from build123d import *

# Parameters (mm, degrees)
ESQUISSE1_W                                        = 65
ESQUISSE1_H                                        = 82
BOSS_EXTRU_1_DEPTH                                 = 10
CHAMBRAGE_POUR_VIS_T_TE_HEXAGONALE_M51_D           = 5.5
CHAMBRAGE_POUR_VIS_T_TE_HEXAGONALE_M51_CBORE_D     = 10
CHAMBRAGE_POUR_VIS_T_TE_HEXAGONALE_M51_CBORE_DEPTH = 7
TROU_TARAUD_M42_D                                  = 3.3
TROU_TARAUD_M42_DEPTH                              = 11.5
TROU_TARAUD_M42_TIP                                = 0.991420021
TROUS_DE_CENTRAGE_4_0MMTRANSITIONAL_1_D            = 4
TROUS_DE_CENTRAGE_4_0MMTRANSITIONAL_1_DEPTH        = 8
TROUS_DE_CENTRAGE_4_0MMTRANSITIONAL_1_TIP          = 1.154700538
TROU_TARAUD_M61_D                                  = 5


with BuildPart() as part:
    # Esquisse1 → Boss.-Extru.1 (new body)
    with BuildSketch(Plane.XY):
        Rectangle(ESQUISSE1_W, ESQUISSE1_H)
    extrude(amount=BOSS_EXTRU_1_DEPTH)

    # Chambrage pour vis à tête hexagonale M51 (through all)
    with Locations(Plane.XY.offset(10)):
        with Locations((10.25, 10), (-9.75, -10)):
            CounterBoreHole(CHAMBRAGE_POUR_VIS_T_TE_HEXAGONALE_M51_D / 2, CHAMBRAGE_POUR_VIS_T_TE_HEXAGONALE_M51_CBORE_D / 2, CHAMBRAGE_POUR_VIS_T_TE_HEXAGONALE_M51_CBORE_DEPTH)

    # Trou taraudé M42
    with Locations(Plane(origin=(32.5, 0, 0), x_dir=(0, 0, -1), z_dir=(1, 0, 0))):
        with Locations((-5, -32), (-5, 32)):
            Hole(TROU_TARAUD_M42_D / 2, depth=TROU_TARAUD_M42_DEPTH)
            with Locations((0, 0, -(TROU_TARAUD_M42_DEPTH + TROU_TARAUD_M42_TIP / 2))):  # 118° drill point
                Cone(0, TROU_TARAUD_M42_D / 2, TROU_TARAUD_M42_TIP, mode=Mode.SUBTRACT)

    # Trous de centrage Ø4.0mmTransitional 1
    with Locations(Plane(origin=(32.5, 0, 0), x_dir=(0, 0, -1), z_dir=(1, 0, 0))):
        with Locations((-5, -19), (-5, 19)):
            Hole(TROUS_DE_CENTRAGE_4_0MMTRANSITIONAL_1_D / 2, depth=TROUS_DE_CENTRAGE_4_0MMTRANSITIONAL_1_DEPTH)
            with Locations((0, 0, -(TROUS_DE_CENTRAGE_4_0MMTRANSITIONAL_1_DEPTH + TROUS_DE_CENTRAGE_4_0MMTRANSITIONAL_1_TIP / 2))):  # 120° drill point
                Cone(0, TROUS_DE_CENTRAGE_4_0MMTRANSITIONAL_1_D / 2, TROUS_DE_CENTRAGE_4_0MMTRANSITIONAL_1_TIP, mode=Mode.SUBTRACT)

    # Trou taraudé M61 (through all)
    with Locations(Plane(origin=(0, 0, 0), x_dir=(-1, 0, 0), z_dir=(0, 0, -1))):
        with Locations((26.5, 28.7), (-24.5, 28.7), (-24.5, -27.3), (26.5, -27.3)):
            Hole(TROU_TARAUD_M61_D / 2)


solid = part.part
Design review of the part built by this model. Coordinates are the model's own, in mm. A direction names the side the tool comes from. Give positions to 0.01 mm unless a question says otherwise; leave off trailing zeros. Loops run counter-clockwise (first coordinate to the right, second up) from the corner with the lowest first, then second, coordinate; pieces in that order, holes last. Notation, with made-up numbers: M 62.5,34 L 86.5,34 A19 ccw 86.5,54 Z; hole C 72.25,-32.5 d11. An arc over 180 degrees is marked long. Answer as a JSON object with one key per item and string values.
Item 1: We need section C-C (z = 8.25). State the section outline as (x, y) points.
Output values:
{"outline": "M -32.5,-41 L 32.5,-41 L 32.5,41 L -32.5,41 Z; hole C -26.5,-27.3 d5; hole C -26.5,28.7 d5; hole C -9.75,-10 d10; hole C 10.25,10 d10; hole C 24.5,-27.3 d5; hole C 24.5,28.7 d5"}
Item 2: We need section D-D (y = -10). State the section outline as (x, z) points, and give its area (4 significant figures).
Output values:
{"outline": "M -32.5,0 L -12.5,0 L -12.5,3 L -14.75,3 L -14.75,10 L -32.5,10 Z; M -7,0 L 32.5,0 L 32.5,10 L -4.75,10 L -4.75,3 L -7,3 Z", "area": "563.5 mm2"}
Item 3: Wall thickness on line 1 along Y through (x, z) = (-27, 6); line 2 along Y through (x, z) = (-9.75, 5); line 3 along Z through (x, y) = (27, 19): over which ranges is each line inside the solid? List them lowest first.
Output values:
{"line 1": "y = -41 to -29.75, -24.85 to 26.25, 31.15 to 41", "line 2": "y = -41 to -15, -5 to 41", "line 3": "z = 0 to 3, 7 to 10"}
Item 4: We need section A-A (y = 28.7). State the section outline as (x, z) points.
Output values:
{"outline": "M -32.5,0 L -29,0 L -29,10 L -32.5,10 Z; M -24,0 L 22,0 L 22,10 L -24,10 Z; M 27,0 L 32.5,0 L 32.5,10 L 27,10 Z"}
Item 5: For P1, Ø4, axis at x = -26.5, y = -27.3, coming from the -Z side; P2, Ø6, axis at x = 10.25, y = 10, coming from the -Z side; P3, Ø8, axis at x = -9.75, y = -10, coming from the +Z side, all flat-tipped, find the tip position at first contact; note any pin that passes through.
Output values:
{"P1": "passes through", "P2": "stops at z = 0", "P3": "stops at z = 3"}
Item 6: Mouldability with a two-part tool opening along Z and no side actions: class faces 1 (the face through (32.5, -1, 5)), 2 (the face through (0, 1, 10)), 3 (the face through (23.546, -19.308, 4.84)) as pulls with the +Z half, pulls with the -Z half, needs draft (parallel to the pull), parting line crosses it, or undercut.
Output values:
{"face 1": "needs draft", "face 2": "pulls with the +Z half", "face 3": "undercut"}
Item 7: We need section B-B (x = 10.25). State the section outline as (y, z) points, and give its area (4 significant figures).
Output values:
{"outline": "M -41,0 L 7.25,0 L 7.25,3 L 5,3 L 5,10 L -41,10 Z; M 12.75,0 L 41,0 L 41,10 L 15,10 L 15,3 L 12.75,3 Z", "area": "733.5 mm2"}
Item 8: Machinability: for faces 4 (the face through (12.4, 7.8, 3)), 5 (the face through (28, -17, 5)), 6 (the face through (-27.04, 26.26, 5.07)), which of the approach directions +Z, -Z, +X, -X, +Y, -Y give a long, thin tool a straight path to every point of the face, cutting with its end or side? Answer none if there is none.
Output values:
{"face 4": "+Z", "face 5": "+X", "face 6": "+Z, -Z"}
